For this review, take the finished solid that the model builds, in its own axes (mm). A direction names the side the tool comes from. Give positions to 0.01 mm unless a question says otherwise; leave off trailing zeros. Write each loop counter-clockwise with the first axis right and the second up, starting at its lowest first coordinate (ties: lowest second). Pieces come first, ordered by that corner, then holes. Notation, with made-up numbers: (67.25, 50) -> (114.25, 50) arc R23 cw to (114.25, 89) -> close; hole circle Ø6 at (58.5, 9.25). An arc over 180 degrees is marked (long way). Answer as CSV lines item,"result".
```python
from build123d import *

# Parameters (mm, degrees)
F0_R     = 4.25
F0_R_2   = 5
F0_R_3   = 10
F1_DEPTH = 5
F2_R     = 5
F2_R_2   = 10
F3_DEPTH = 2


with BuildPart() as f1:
    # F0 (on Top) → F1 (new body)
    with BuildSketch(Plane.XY):
        with BuildLine():
            Line((-10, 40), (-115, 40))
            Line((-115, 40), (-115, -40))
            Line((-115, -40), (115, -40))
            Line((115, -40), (115, 40))
            Line((115, 40), (10, 40))
            Line((10, 40), (10, 35))
            ThreePointArc((10, 35), (0, 25), (-10, 35))
            Line((-10, 35), (-10, 40))
        make_face()
        with Locations((-105, -30)):
            Circle(F0_R, mode=Mode.SUBTRACT)
        with Locations((105, -30)):
            Circle(F0_R, mode=Mode.SUBTRACT)
        with Locations((-35, 0)):
            Circle(F0_R_2, mode=Mode.SUBTRACT)
        with Locations((-105, 30)):
            Circle(F0_R, mode=Mode.SUBTRACT)
        Circle(F0_R_3, mode=Mode.SUBTRACT)
        with Locations((35, 0)):
            Circle(F0_R_2, mode=Mode.SUBTRACT)
        with Locations((105, 30)):
            Circle(F0_R, mode=Mode.SUBTRACT)
    extrude(amount=F1_DEPTH)

    # F2 (on face) → F3 (cut)
    with BuildSketch(Plane.XY.offset(5)):
        with Locations((-35, 0)):
            Circle(F2_R)
        with Locations((35, 0)):
            Circle(F2_R)
        with Locations((35, 0)):
            Circle(F2_R_2)
        with Locations((35, 0)):
            Circle(F2_R, mode=Mode.SUBTRACT)
        with Locations((-35, 0)):
            Circle(F2_R_2)
        with Locations((-35, 0)):
            Circle(F2_R, mode=Mode.SUBTRACT)
    extrude(amount=-F3_DEPTH, mode=Mode.SUBTRACT)


solid = f1.part
```
Q1. Add section C-C (x = 105). Write out the cut boundary in (y, z), plus the area to 3 significant figures.
Answer block:
outline,"(-40, 0) -> (-34.25, 0) -> (-34.25, 5) -> (-40, 5) -> close; (-25.75, 0) -> (25.75, 0) -> (25.75, 5) -> (-25.75, 5) -> close; (34.25, 0) -> (40, 0) -> (40, 5) -> (34.25, 5) -> close"
area,"315 mm2"
Q2. Draft analysis for pull direction X (two halves, no side actions). For faces 4 (the cylindrical face through (-109.246, -29.813, 2.465)), 5 (the flat face through (30, -2, 3)), 6 (the flat face through (115, -1, 2)), 7 (the flat face through (-2, -17, 0)), state which applies: released by +X, released by -X, zero draft, split by the parting line, or undercut.
Answer block:
face 4,"undercut"
face 5,"undercut"
face 6,"released by +X"
face 7,"zero draft"
Q3. Add section B-B (x = 35). Write out the cut boundary in (y, z).
Answer block:
outline,"(-40, 0) -> (-5, 0) -> (-5, 3) -> (-10, 3) -> (-10, 5) -> (-40, 5) -> close; (5, 0) -> (40, 0) -> (40, 5) -> (10, 5) -> (10, 3) -> (5, 3) -> close"
Q4. Add section D-D (z = 4.05). Write out the cut boundary in (x, y).
Answer block:
outline,"(-115, -40) -> (115, -40) -> (115, 40) -> (10, 40) -> (10, 35) arc R10 cw to (-10, 35) -> (-10, 40) -> (-115, 40) -> close; hole circle Ø8.5 at (-105, -30); hole circle Ø8.5 at (-105, 30); hole circle Ø20 at (-35, 0); hole circle Ø20 at (0, 0); hole circle Ø20 at (35, 0); hole circle Ø8.5 at (105, -30); hole circle Ø8.5 at (105, 30)"
Q5. For faces 1 (the flat face through (-10, 37, 2)), 2 (the flat face through (-2, -40, 2)), 3 (the cylindrical face through (-45, 0, 4)), list the 3-axis set-ups (+Z, -Z, +X, -X, +Y, -Y) from which the entire face can be reached by the end or side of a thin tool; tool diameter is ignored.
Answer block:
face 1,"+Z, -Z, +Y"
face 2,"+Z, -Z, +X, -X, -Y"
face 3,"+Z"
Q6. Clearance check with flat-ended pins moving along their axes: pin 1 (8 mm diameter, centred on x = -36, y = -25, fed in from -Z); pin 2 (6 mm diameter, centred on x = 31, y = 0.5, fed in from +Z). State where each tip first meets the part, or that it passes through.
Answer block:
pin 1,"stops at z = 0"
pin 2,"stops at z = 3"
Q7. To check wall thickness, follow probe 1 along Y at (x, z) = (-105, 3.7); probe 2 along X at (y, z) = (33, 3.15); probe 3 along Y at (x, z) = (-35, 0.8). State the ranges of each line that lie inside material, in increasing order. Write a range as [from, to].
Answer block:
probe 1,"y = [-40, -34.25], [-25.75, 25.75], [34.25, 40]"
probe 2,"x = [-115, -108.01], [-101.99, -9.8], [9.8, 101.99], [108.01, 115]"
probe 3,"y = [-40, -5], [5, 40]"
Q8. Add section A-A (y = -30). Write out the cut boundary in (x, z).
Answer block:
outline,"(-115, 0) -> (-109.25, 0) -> (-109.25, 5) -> (-115, 5) -> close; (-100.75, 0) -> (100.75, 0) -> (100.75, 5) -> (-100.75, 5) -> close; (109.25, 0) -> (115, 0) -> (115, 5) -> (109.25, 5) -> close"
